Can you work these out from the model? Positions are in its coordinate system, mm. Face numbers are marked on the shaded views. A direction names the side the tool comes from. Round coordinates to 2 decimals unless told otherwise and drop trailing zeros. Write each loop counter-clockwise with the first axis right and the second up, starting at its lowest first coordinate (ties: lowest second). Pieces come first, ordered by that corner, then holes.
Q1. If we section it at A-A (y = 0): Please give me the cut outline in (x, z).
Q2. If we section it at C-C (x = 128): Please give me the cut outline in (y, z), plus the area to 3 significant figures.
Q3. I'm going to push flat-ended pins straight in: pin 1 Ø2 at (y, z) = (12.5, 48.5) entering from -X; pin 2 Ø2 at (x, y) = (217.5, -16.5) entering from -Z; pin 3 Ø8 at (y, z) = (26, 32) entering from -X. Where does each tip first touch, or does it pass through?
Q4. If we section it at B-B (z = 93.5): Please give me the cut outline in (x, y).
Q5. For the marked faces 1 and 2, which set-ups out of +Z, -Z, +X, -X, +Y, -Y let a thin tool reach every point of the face, with its end or its side?
Q6. Please list where these lines run through material, in increasing order: line 1 along Z through (x, y) = (127.5, -18.5); line 2 along X through (y, z) = (2, 34.5); line 3 along Z through (x, y) = (87, -13).
Q7. If we section it at D-D (y = -17): Please give me the cut outline in (x, z), plus the area to 3 significant figures.
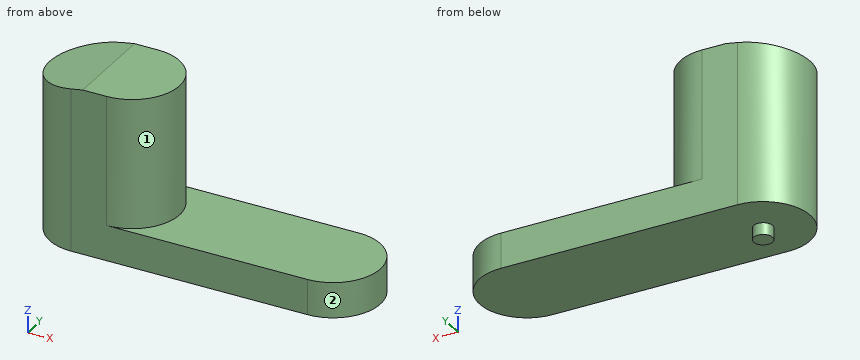
Autodesk Inventor part; units mm, degrees
ref_plane "YZ Plane" through (0, 0, 0) normal (1, 0, 0) x (0, 1, 0)
ref_plane "XZ Plane" through (0, 0, 0) normal (0, 1, 0) x (-1, 0, 0)
ref_plane "XY Plane" through (0, 0, 0) normal (0, 0, 1) x (1, 0, 0)
sketch "Sketch1" plane through (0, 0, 0) normal (0, 0, 1) x (1, 0, 0)
  line L0 (0, 15.9441) -> (0, -15.9441) construction
  line L1 (11.6084, 0) -> (-11.6084, 0) construction
  line L2 (46.4051, 40) -> (246.4051, 40)
  line L3 (246.4051, 40) -> (246.4051, -40)
  line L4 (246.4051, -40) -> (46.4051, -40)
  line L5 (46.4051, -40) -> (46.4051, 40)
  circle A0 centre (46.4051, 0) radius 40
  circle A1 centre (246.4051, 0) radius 40
  point P0 (0, 0)
  point P1 (0, 0)
  dimension "d0" = 80
  dimension "d1" = 200
extrude "Extrusion1" add sketch "Sketch1" along normal blind 30
sketch "Sketch2" plane through (0, 0, 30) normal (0, 0, 1) x (1, 0, 0)
  arc A0 (46.4051, 40) -> (46.4051, -40) centre (46.4051, 0) ccw
  circle A1 centre (46.4051, 0) radius 40
  line L0 (46.4051, -40) -> (46.4051, 40)
  line L1 (116.4051, 0) -> (76.4051, 0)
  circle A2 centre (76.4051, 0) radius 40
  line L2 (46.4051, 40) -> (76.4051, 40)
  line L3 (76.4051, -40) -> (46.4051, -40)
  point P0 (0, 0)
extrude "Extrusion2" add sketch "Sketch2" along normal blind 110
sketch "Sketch3" plane through (46.4051, -40, 0) normal (0, -1, 0) x (1, 0, 0)
  line L0 (-40, 140) -> (0, 140)
  line L1 (0, 140) -> (10, 140)
  line L2 (10, 140) -> (-81.693, 123.8321)
  line L3 (-81.693, 123.8321) -> (-81.693, 140)
  line L4 (-81.693, 140) -> (0, 140)
  point P0 (-46.4051, 0)
extrude "Extrusion3" cut sketch "Sketch3" against normal through all
sketch "Sketch4" plane through (0, 0, 0) normal (0, 0, -1) x (-1, 0, 0)
  line L0 (-246.4051, -40) -> (-46.4051, -40)
  arc A0 (-46.4051, -40) -> (-46.4051, 40) centre (-46.4051, 0) ccw
  line L1 (-46.4051, 40) -> (-246.4051, 40)
  arc A1 (-246.4051, 40) -> (-246.4051, -40) centre (-246.4051, 0) ccw
  circle A2 centre (-46.4051, 0) radius 8
  point P0 (0, 0)
extrude "Extrusion4" add sketch "Sketch4" along normal blind 10 contours A2
properties part number "CANH TAY 3"
A:
1. outline: (6.41, 0) - (38.41, 0) - (38.41, -10) - (54.41, -10) - (54.41, 0) - (286.41, 0) - (286.41, 30) - (116.41, 30) - (116.41, 140) - (56.41, 140) - (6.41, 131.18) - close
2. outline: (-40, 0) - (40, 0) - (40, 30) - (-40, 30) - close
2. area: 2,400 mm2
3. pin 1: stops at x = 8.09
3. pin 2: stops at z = 0
3. pin 3: stops at x = 13
4. outline: (46.41, -40) - (76.41, -40) arc R40 ccw to (76.41, 40) - (46.41, 40) arc R40 ccw to start
5. face 1: +Z, +X
5. face 2: +Z, -Z, +X
6. line 1: z = 0 to 30
6. line 2: x = 6.46 to 116.36
6. line 3: z = 0 to 140
7. outline: (10.2, 0) - (282.61, 0) - (282.61, 30) - (112.61, 30) - (112.61, 140) - (56.41, 140) - (10.2, 131.85) - close
7. area: 19,200 mm2
